The model under review builds one solid part; all positions refer to its coordinate system, in mm. Give positions to 0.01 mm unless a question says otherwise; leave off trailing zeros. Write each loop counter-clockwise with the first axis right and the second up, starting at its lowest first coordinate (ties: lowest second). Pieces come first, ordered by that corner, then holes. Notation, with made-up numbers: (-32.75, -35) - (3.25, -35) arc R26 cw to (3.25, -16) - close; hole circle Ø5 at (-27, 38). An arc over 180 degrees is marked (long way). One line per question, with ' | ' between items. Start each with the question number.
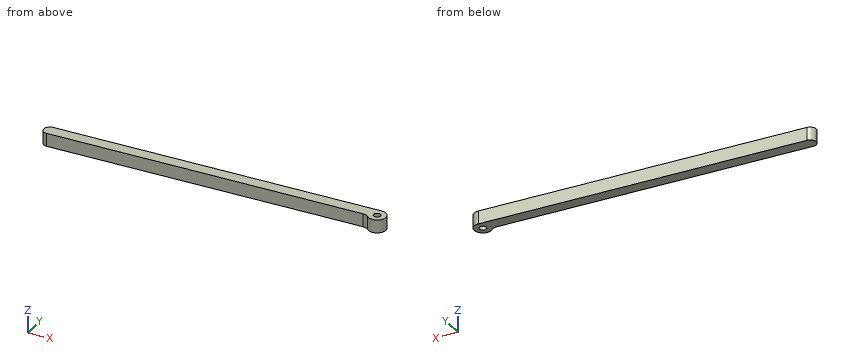
Autodesk Inventor part; units mm, degrees
ref_plane "YZ Plane" through (0, 0, 0) normal (1, 0, 0) x (0, 1, 0)
ref_plane "XZ Plane" through (0, 0, 0) normal (0, 1, 0) x (-1, 0, 0)
ref_plane "XY Plane" through (0, 0, 0) normal (0, 0, 1) x (1, 0, 0)
ref_plane "Work Plane1" through (0, 0, 0) normal (0, 0, 1) x (1, 0, 0)
sketch "Sketch1" plane through (0, 0, 0) normal (0, 0, 1) x (1, 0, 0)
  circle A0 centre (77.9, 1) radius 0.8
  line L0 (79.585, 1.6) -> (78.4292, 1.6) construction
  line L1 (2.9, 3) -> (77.9, 3)
  arc A1 (2.9, 3) -> (2.9, 0.2) centre (2.9, 1.6) ccw
  arc A2 (76.4, -0.3229) -> (77.9, 3) centre (77.9, 1) ccw
  line L2 (75.0516, 0.2) -> (2.9, 0.2)
  arc A3 (76.4, -0.3229) -> (75.0516, 0.2) centre (75.0516, -1.8) ccw
  point P0 (0, 0)
  point P1 (41.1836, 1.6)
  point P2 (74.7858, 0.2)
  dimension "d1" = 4
  dimension "d2" = 2.8
  dimension "d4" = 2
  dimension "d5" = 75
  dimension "d6" = 1.5
extrude "Extrusion1" add sketch "Sketch1" along normal blind 3
properties part number "flip-stand-bottom"
Item 1: Clearance check with a flat-ended pin moving along its axis: P1, Ø1, axis at x = 40.5, z = 2, coming from the -Y side. State where the tip first meets the part, or that it passes through.
Item 2: For probe 1 along Y at (x, z) = (77.9, 0.8); probe 2 along Y at (x, z) = (54, 1.5); probe 3 along X at (y, z) = (1.2, 2.5), list the stretches that pass through material, from the lowest coordinate up.
Item 3: Take a section at B-B (y = 1). Give the boundary of the cut face in (x, z), plus the area to 3 significant figures.
Item 4: Take a section at C-C (x = 67.5). Give the boundary of the cut face in (y, z), plus the area to 3 significant figures.
Item 5: Take a section at A-A (z = 1.9). Give the boundary of the cut face in (x, y).
Check sheet entries:
1) P1: stops at y = 0.2
2) probe 1: y = -1 to 0.2, 1.8 to 3 | probe 2: y = 0.2 to 3 | probe 3: x = 1.56 to 77.13, 78.67 to 79.89
3) outline: (1.64, 0) - (77.1, 0) - (77.1, 3) - (1.64, 3) - close; (78.7, 0) - (79.9, 0) - (79.9, 3) - (78.7, 3) - close | area: 230 mm^2
4) outline: (0.2, 0) - (3, 0) - (3, 3) - (0.2, 3) - close | area: 8.40 mm^2
5) outline: (2.9, 0.2) - (75.05, 0.2) arc R2 cw to (76.4, -0.32) arc R2 ccw (long way) to (77.9, 3) - (2.9, 3) arc R1.4 ccw to start; hole circle Ø1.6 at (77.9, 1)
